from build123d import *

# Parameters (mm, degrees)
BASE_FLANGE1_DEPTH   = 165.1
SKETCH6_W            = 63.5
SKETCH6_H            = 38.1
CUT_EXTRUDE1_DEPTH   = 218.169427211
CHAMFER1_SIZE        = 2.54
SKETCH8_R            = 2.54
BOSS_EXTRUDE1_DEPTH  = 10.7315
LPATTERN1_COUNT      = 2
LPATTERN1_PITCH      = 31.75
LPATTERN1_COUNT_DIR2 = 2
LPATTERN1_PITCH_DIR2 = 86.106
SKETCH9_R            = 3.969000063
CUT_EXTRUDE2_DEPTH   = 218.169427211
LPATTERN2_COUNT      = 2
LPATTERN2_PITCH      = 19.05
CUT_EXTRUDE3_DEPTH   = 218.169427211
CUT_EXTRUDE5_REACH   = 228.091
SKETCH11_R           = 1.5875
SKETCH11_W           = 72
SKETCH11_H           = 21.2
SKETCH12_R           = 1.5875
CUT_EXTRUDE6_DEPTH   = 3
SKETCH13_R           = 1.234202105
SKETCH13_W           = 16.55
SKETCH13_H           = 14.55
CUT_EXTRUDE7_DEPTH   = 3
FILLET1_R            = 1.3
FILLET2_R            = 1.27
SKETCH14_R           = 1.4224
CUT_EXTRUDE8_DEPTH   = 6.35


# Sheet-metal steps are written as plain solids
with BuildPart() as part:
    # Sketch1 → Base-Flange1 (new body)
    with BuildSketch(Plane(origin=(0, 0, 0), x_dir=(0, 0, -1), z_dir=(1, 0, 0))):
        with BuildLine():
            Line((21.322905549, 20.238293522), (21.322905549, 14.71329365))
            ThreePointArc((21.322905549, 14.71329365), (22.494478461, 11.884866435), (25.322905677, 10.713293522))
            Line((25.322905677, 10.713293522), (60.310580797, 10.713293522))
            ThreePointArc((60.310580797, 10.713293522), (71.985098111, 16.15721035), (75.319050953, 28.59969175))
            Line((75.319050953, 28.59969175), (58.299970775, 125.11969175))
            ThreePointArc((58.299970775, 125.11969175), (53.087583791, 134.147810835), (43.291500619, 137.713293522))
            Line((43.291500619, 137.713293522), (25.322905677, 137.713293522))
            ThreePointArc((25.322905677, 137.713293522), (22.494478461, 136.541720609), (21.322905549, 133.713293394))
            Line((21.322905549, 133.713293394), (21.322905549, 128.188293522))
            Line((21.322905549, 128.188293522), (18.322905549, 128.188293522))
            Line((18.322905549, 128.188293522), (18.322905549, 133.713293394))
            ThreePointArc((18.322905549, 133.713293394), (20.373158118, 138.663040953), (25.322905677, 140.713293522))
            Line((25.322905677, 140.713293522), (43.291500619, 140.713293522))
            ThreePointArc((43.291500619, 140.713293522), (55.01594662, 136.445944164), (61.254394034, 125.640636283))
            Line((61.254394034, 125.640636283), (78.273474212, 29.120636283))
            ThreePointArc((78.273474212, 29.120636283), (74.28323144, 14.228847521), (60.310580797, 7.713293522))
            Line((60.310580797, 7.713293522), (25.322905677, 7.713293522))
            ThreePointArc((25.322905677, 7.713293522), (20.373158118, 9.763546091), (18.322905549, 14.71329365))
            Line((18.322905549, 14.71329365), (18.322905549, 20.238293522))
            Line((18.322905549, 20.238293522), (21.322905549, 20.238293522))
        make_face()
    extrude(amount=BASE_FLANGE1_DEPTH)

    # Sketch6 → Cut-Extrude1 (cut, through all)
    with BuildSketch(Plane(origin=(0, 14.263647062, -80.893162264), x_dir=(-1, 0, 0), z_dir=(0, 0.1736481776669347, -0.9848077530122075))):
        with Locations((-67.564, 68.645158806)):
            Rectangle(SKETCH6_W, SKETCH6_H)
    extrude(amount=-CUT_EXTRUDE1_DEPTH, mode=Mode.SUBTRACT)

    # Chamfer1
    chamfer1_edges = [part.edges().sort_by_distance(p)[0] for p in [
        (99.314, 81.865931661, -68.973055532),
        (67.564, 63.105343966, -72.281053316),
        (35.814, 81.865931661, -68.973055532),
        (67.564, 100.626519356, -65.665057747),
    ]]
    chamfer(chamfer1_edges, length=CHAMFER1_SIZE)

    # Sketch8 → Boss-Extrude1 (add)
    with BuildSketch(Plane(origin=(0, 13.742702529, -77.938739005), x_dir=(1, 0, 0), z_dir=(0, -0.1736481776669347, 0.9848077530122075))):
        with Locations(Location((25.4, 49.595158806, 0), (0, 0, 270))):
            Circle(SKETCH8_R)
    boss_extrude1 = extrude(amount=BOSS_EXTRUDE1_DEPTH)

    # LPattern1: Boss-Extrude1 2 × 2
    with Locations(*[Vector(0, 0.9848077530122074, 0.17364817766693458) * (i * LPATTERN1_PITCH) + Vector(1, 0, 0) * (j * LPATTERN1_PITCH_DIR2) for i in range(LPATTERN1_COUNT) for j in range(LPATTERN1_COUNT_DIR2) if (i, j) != (0, 0)]):
        add(boss_extrude1)

    # Sketch9 → Cut-Extrude2 (cut, through all)
    with BuildSketch(Plane(origin=(0, 14.263647062, -80.893162264), x_dir=(-1, 0, 0), z_dir=(0, 0.1736481776669347, -0.9848077530122075))):
        with Locations(Location((-52.3748, 25.312758806, 0), (0, 0, 90))):
            Circle(SKETCH9_R)
    cut_extrude2 = extrude(amount=-CUT_EXTRUDE2_DEPTH, mode=Mode.SUBTRACT)

    # LPattern2: Cut-Extrude2 ×2
    with Locations(*[(-i * LPATTERN2_PITCH, 0, 0) for i in range(1, LPATTERN2_COUNT)]):
        add(cut_extrude2, mode=Mode.SUBTRACT)

    # Sketch10 → Cut-Extrude3 (cut, through all)
    with BuildSketch(Plane(origin=(0, 14.263647062, -80.893162264), x_dir=(-1, 0, 0), z_dir=(0, 0.17364817766693483, -0.9848077530122072))):
        with BuildLine():
            Line((-147.577626964, 39.365158806), (-147.577626964, 36.965158806))
            Line((-147.577626964, 36.965158806), (-146.505365759, 36.965158806))
            ThreePointArc((-146.505365759, 36.965158806), (-126.577626964, 38.165158806), (-146.505365759, 39.365158806))
            Line((-146.505365759, 39.365158806), (-147.577626964, 39.365158806))
        make_face()
    extrude(amount=-CUT_EXTRUDE3_DEPTH, mode=Mode.SUBTRACT)

    # Sketch11 → Cut-Extrude5 (cut, up to next)
    with BuildSketch(Plane(origin=(0, 7.713293522, 0), x_dir=(-1, 0, 0), z_dir=(0, -1, 0)), mode=Mode.PRIVATE) as cut_extrude5_sk1:
        with Locations(Location((-41.25, 38.327705677, 0), (0, 0, 90))):
            Circle(SKETCH11_R)
    cut_extrude5_tool1 = extrude(cut_extrude5_sk1.sketch, amount=-CUT_EXTRUDE5_REACH, mode=Mode.PRIVATE) & part.part
    # Sketch11 → Cut-Extrude5 (cut, up to next)
    with BuildSketch(Plane(origin=(0, 7.713293522, 0), x_dir=(-1, 0, 0), z_dir=(0, -1, 0)), mode=Mode.PRIVATE) as cut_extrude5_sk2:
        with Locations(Location((-123.85, 38.327705677, 0), (0, 0, 90))):
            Circle(SKETCH11_R)
    cut_extrude5_tool2 = extrude(cut_extrude5_sk2.sketch, amount=-CUT_EXTRUDE5_REACH, mode=Mode.PRIVATE) & part.part
    # Sketch11 → Cut-Extrude5 (cut, up to next)
    with BuildSketch(Plane(origin=(0, 7.713293522, 0), x_dir=(-1, 0, 0), z_dir=(0, -1, 0)), mode=Mode.PRIVATE) as cut_extrude5_sk3:
        with Locations((-82.55, 38.327705677)):
            Rectangle(SKETCH11_W, SKETCH11_H)
    cut_extrude5_tool3 = extrude(cut_extrude5_sk3.sketch, amount=-CUT_EXTRUDE5_REACH, mode=Mode.PRIVATE) & part.part
    add(cut_extrude5_tool1.solids().sort_by_distance((41.25, 7.713294, -38.327706))[0], mode=Mode.SUBTRACT)
    add(cut_extrude5_tool2.solids().sort_by_distance((123.85, 7.713294, -38.327706))[0], mode=Mode.SUBTRACT)
    add(cut_extrude5_tool3.solids().sort_by_distance((82.55, 7.713294, -38.327706))[0], mode=Mode.SUBTRACT)

    # Sketch12 → Cut-Extrude6 (cut)
    with BuildSketch(Plane.XY.offset(-18.322905549)):
        with Locations((152.4, 130.950793458)):
            Circle(SKETCH12_R)
        with Locations((152.4, 17.475793586)):
            Circle(SKETCH12_R)
        with Locations((82.55, 17.475793586)):
            Circle(SKETCH12_R)
        with Locations((82.55, 130.950793458)):
            Circle(SKETCH12_R)
        with Locations((12.7, 130.950793458)):
            Circle(SKETCH12_R)
        with Locations((12.7, 17.475793586)):
            Circle(SKETCH12_R)
    extrude(amount=-CUT_EXTRUDE6_DEPTH, mode=Mode.SUBTRACT)

    # Sketch13 → Cut-Extrude7 (cut)
    with BuildSketch(Plane(origin=(0, 7.713293522, 0), x_dir=(-1, 0, 0), z_dir=(0, -1, 0))):
        with Locations(Location((-3.24, 35.61403221, 0), (0, 0, 90))):
            Circle(SKETCH13_R)
        with Locations(Location((-27.24, 44.61403221, 0), (0, 0, 90))):
            Circle(SKETCH13_R)
        with Locations((-15.24, 40.11403221)):
            Rectangle(SKETCH13_W, SKETCH13_H)
    extrude(amount=-CUT_EXTRUDE7_DEPTH, mode=Mode.SUBTRACT)

    # Fillet1
    fillet1_edges = [part.edges().sort_by_distance(p)[0] for p in [
        (6.965, 9.213293522, -47.38903221),
        (6.965, 9.213293522, -32.83903221),
        (23.515, 9.213293522, -32.83903221),
        (23.515, 9.213293522, -47.38903221),
    ]]
    fillet(fillet1_edges, radius=FILLET1_R)

    # Fillet2
    fillet2_edges = [part.edges().sort_by_distance(p)[0] for p in [
        (52.3748, 35.283146151, -77.186857454),
        (33.3248, 35.283146151, -77.186857454),
    ]]
    fillet(fillet2_edges, radius=FILLET2_R)

    # Sketch14 → Cut-Extrude8 (cut)
    with BuildSketch(Plane(origin=(0, 11.87919711, -67.370274604), x_dir=(1, 0, 0), z_dir=(0, -0.17364817766693477, 0.9848077530122074))):
        with Locations(Location((111.506, 81.345158806, 0), (0, 0, 270))):
            Circle(SKETCH14_R)
        with Locations(Location((111.506, 49.595158806, 0), (0, 0, 270))):
            Circle(SKETCH14_R)
        with Locations(Location((25.4, 49.595158806, 0), (0, 0, 270))):
            Circle(SKETCH14_R)
        with Locations(Location((25.4, 81.345158806, 0), (0, 0, 270))):
            Circle(SKETCH14_R)
    extrude(amount=-CUT_EXTRUDE8_DEPTH, mode=Mode.SUBTRACT)


solid = part.part
Read the model definition and answer for the solid it produces. Units are mm, in the model's axes. A direction names the side the tool comes from. Coordinates: 2 decimals unless noted, no trailing zeros. Order: outer loops, then holes, each group sorted by start corner. A loop starts at its lowest first (then second) coordinate and runs counter-clockwise, first axis right, second up. Notation, with made-up numbers: M 20,-39.75 L 39,-39.75 A17 cw 39,-10.75 Z; hole C 19.25,10.25 d9. An arc over 180 degrees is marked long. Put each result on its own line as item: value. Start each with the question number.
Item 1: The mould has two halves that part along X. Classify faces 5 (the face through (34.56, 81.34, -67.76)), 6 (the face through (0, 70, -69)), 7 (the face through (81, 137.713, -34)): +X half, -X half, draft (parallel to the pull), parting line (faces both ways), or undercut.
Item 2: Consider probe 1 along Y at (x, z) = (12.7, -20.5); probe 2 along Y at (x, z) = (74, -27.5); probe 3 along Y at (x, z) = (82.55, -19.15). Determine where each line is inside the solid, lowest interval first. Write a range as [from, to].
Item 3: Given pin 1 Ø12 at (x, y) = (66.5, 59.5) entering from +Z; pin 2 Ø3 at (x, y) = (12.7, 17.48) entering from -Z (3 decimals); pin 3 Ø2.5 at (x, y) = (17, 8.5) entering from +Z, each flat-ended and moving along its own axis, determine where each tip first touches the part or whether it passes through.
Item 4: Section A-A, the plane x = 78.5 is taken. Count the separate pieces of the cut face and the enclosed holes in it, plus the area to 3 significant figures.
Item 5: For faces 1 (the face through (26.6, 60.51, -61.97)), 2 (the face through (35.814, 81.1, -66.3)), 3 (the face through (23.74, 60.76, -58.75)), 4 (the face through (81.39, 11.92, -22.46)), determine the directions among +Z, -Z, +X, -X, +Y, -Y from which every point of the face is accessible in a straight line to the end or side of a thin tool.
Item 6: Section B-B, the plane y = 117 is taken. Determine the outline of the cut face in (x, z), plus the area to 3 significant figures.
Computed:
1. face 5: undercut
1. face 6: -X half
1. face 7: draft
2. probe 1: y = [9.64, 15.89], [19.06, 20.24], [128.19, 129.36], [132.54, 138.79]
2. probe 2: y = [7.71, 10.71], [137.71, 140.71]
2. probe 3: y = [11.41, 15.89], [19.06, 20.24], [128.19, 129.36], [132.54, 137.01]
3. pin 1: stops at z = -69.33
3. pin 2: stops at z = -77.165
3. pin 3: stops at z = -20.39
4. separate pieces: 3
4. enclosed holes: 0
4. area: 511 mm2
5. face 1: none
5. face 2: +Z, -Z
5. face 3: +Z, +X, -X
5. face 4: +X, -X
6. outline: M 0,-62.78 L 165.1,-62.78 L 165.1,-59.73 L 0,-59.73 Z
6. area: 503 mm2
